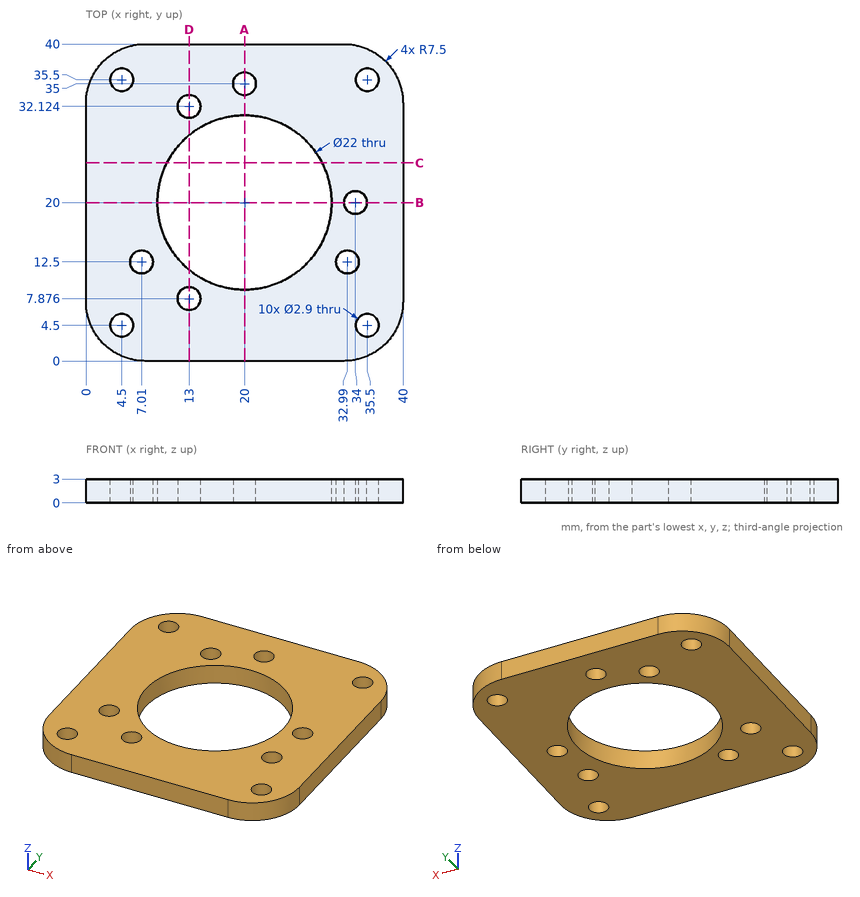
The drawing under review shows one solid part. Ordinate dimensions are in mm from its lowest x, y, z. Give positions to 0.01 mm unless a question says otherwise; leave off trailing zeros. Loops run counter-clockwise (first coordinate to the right, second up) from the corner with the lowest first, then second, coordinate; pieces in that order, holes last. Notation, with made-up numbers: M 71.5,72 L 91.5,72 A27 cw 91.5,96 Z; hole C 25.5,30 d6. An arc over 180 degrees is marked long. One line per question, with ' | ' between items. Start each with the question number.
1. Insertion check: P1, Ø2.5, axis at x = 20, y = 35, coming from the -Z side. The pin has a flat end and moves straight along its axis. Give the tip position at first contact, or say it passes through.
2. Add section C-C (y = 25). Write out the cut boundary in (x, z).
3. Add section A-A (x = 20). Write out the cut boundary in (y, z), plus the area to 3 significant figures.
4. Add section B-B (y = 20). Write out the cut boundary in (x, z), plus the area to 3 significant figures.
5. To check wall thickness, follow L1, parallel to X at y = 20, z = 1.05; L2, parallel to Y at x = 20, z = 1.65; L3, parallel to Y at x = 36, z = 0.95. State the ranges of each line that lie inside material, in increasing order.
6. Add section D-D (x = 13). Write out the cut boundary in (y, z) (1 decimal).
Worked out:
1) P1: passes through
2) outline: M 0,0 L 10.2,0 L 10.2,3 L 0,3 Z; M 29.8,0 L 40,0 L 40,3 L 29.8,3 Z
3) outline: M 0,0 L 9,0 L 9,3 L 0,3 Z; M 31,0 L 33.55,0 L 33.55,3 L 31,3 Z; M 36.45,0 L 40,0 L 40,3 L 36.45,3 Z | area: 45.3 mm²
4) outline: M 0,0 L 9,0 L 9,3 L 0,3 Z; M 31,0 L 32.55,0 L 32.55,3 L 31,3 Z; M 35.45,0 L 40,0 L 40,3 L 35.45,3 Z | area: 45.3 mm²
5) L1: x = 0 to 9, 31 to 32.55, 35.45 to 40 | L2: y = 0 to 9, 31 to 33.55, 36.45 to 40 | L3: y = 0.87 to 3.14, 5.86 to 34.14, 36.86 to 39.13
6) outline: M 0,0 L 6.4,0 L 6.4,3 L 0,3 Z; M 9.3,0 L 11.5,0 L 11.5,3 L 9.3,3 Z; M 28.5,0 L 30.7,0 L 30.7,3 L 28.5,3 Z; M 33.6,0 L 40,0 L 40,3 L 33.6,3 Z
